```python
from build123d import *

# Parameters (mm, degrees)
F0_W     = 120
F0_H     = 120
F0_R     = 9
F1_DEPTH = 12
F2_SIZE  = 0.5


with BuildPart() as f1:
    # F0 (on Top) → F1 (new body)
    with BuildSketch(Plane.XY):
        Rectangle(F0_W, F0_H)
        Circle(F0_R, mode=Mode.SUBTRACT)
    extrude(amount=F1_DEPTH)

    # F2
    f2_edges = [f1.edges().sort_by_distance(p)[0] for p in [
        (9, 0, 6),
        (-9, 0, 0),
        (-9, 0, 12),
    ]]
    chamfer(f2_edges, length=F2_SIZE)


solid = f1.part
```
Build history of the part. All positions in model axes, mm. Round coordinates to 2 decimals unless told otherwise and drop trailing zeros. Loops run counter-clockwise (first coordinate to the right, second up) from the corner with the lowest first, then second, coordinate; pieces in that order, holes last.
Item 1: Saw through at A-A (x = 0). List the corners of the cut face in (y, z), then the cut area to 3 significant figures.
Item 2: Two-plate mould, pull along Y, no slides. Class faces 1 (the face through (-1.172, 8.923, 5.923)), 2 (the face through (-1, 60, 6)), 3 (the face through (-14, 1, 0)): released by +Y, released by -Y, zero draft, split by the parting line, or undercut.
Item 3: Saw through at B-B (z = 9.5). List the corners of the cut face in (x, y).
Item 4: Drill centre lines: line 1 along Y through (x, z) = (0, 6); line 2 along X through (y, z) = (-6.5, 7.5); line 3 along Y through (x, z) = (-1, 4). Where is each one in solid material? Low to high.
Worked answers:
1. outline: (-60, 0) - (-9.5, 0) - (-9, 0.5) - (-9, 11.5) - (-9.5, 12) - (-60, 12) - close; (9, 0.5) - (9.5, 0) - (60, 0) - (60, 12) - (9.5, 12) - (9, 11.5) - close
1. area: 1,220 mm2
2. face 1: undercut
2. face 2: released by +Y
2. face 3: zero draft
3. outline: (-60, -60) - (60, -60) - (60, 60) - (-60, 60) - close; hole circle Ø18 at (0, 0)
4. line 1: y = -60 to -9, 9 to 60
4. line 2: x = -60 to -6.22, 6.22 to 60
4. line 3: y = -60 to -8.94, 8.94 to 60
